Can you work these out from the model? Positions are in its coordinate system, mm. A direction names the side the tool comes from. Give positions to 0.01 mm unless a question says otherwise; leave off trailing zeros. Loops run counter-clockwise (first coordinate to the right, second up) from the corner with the lowest first, then second, coordinate; pieces in that order, holes last. Notation, with made-up numbers: M 56.25,-37 L 80.25,-37 A22 ccw 80.25,2 Z; hole C -0.5,-1 d5. An arc over 180 degrees is marked long. Answer as a JSON object with one key per item and string values.
```python
from build123d import *

# Parameters (mm, degrees)
F1_DEPTH = 120
F3_DEPTH = 1.001


# Not quite as in the source:
# - a feature names something its author has since deleted; it is built from what else it names


with BuildPart() as f1:
    # F0 (on Front) → F1 (new body)
    with BuildSketch(Plane.XZ):
        Polygon((-17.5, 6), (-17.5, 5), (-13.5, 5), (-13.5, -1), (13.5, -1), (13.5, 5), (17.5, 5), (17.5, 6), (12.5, 6), (12.5, 0), (-12.5, 0), (-12.5, 6), align=None)
    extrude(amount=F1_DEPTH)

    # F2 (on face) → F3 (cut, through all)
    with BuildSketch(Plane.XY):
        with BuildLine():
            ThreePointArc((-2.25, -28.25), (0, -30.5), (2.25, -28.25))
            Line((2.25, -28.25), (2.25, -7.75))
            ThreePointArc((2.25, -7.75), (0, -5.5), (-2.25, -7.75))
            Line((-2.25, -7.75), (-2.25, -28.25))
        make_face()
        with BuildLine():
            Line((-2.25, -43.75), (-2.25, -64.25))
            ThreePointArc((-2.25, -64.25), (0, -66.5), (2.25, -64.25))
            Line((2.25, -64.25), (2.25, -43.75))
            ThreePointArc((2.25, -43.75), (0, -41.5), (-2.25, -43.75))
        make_face()
        with BuildLine():
            Line((-2.25, -79.75), (-2.25, -100.25))
            ThreePointArc((-2.25, -100.25), (0, -102.5), (2.25, -100.25))
            Line((2.25, -100.25), (2.25, -79.75))
            ThreePointArc((2.25, -79.75), (0, -77.5), (-2.25, -79.75))
        make_face()
        with BuildLine():
            Line((-2.25, -120), (-2.25, -136.25))
            ThreePointArc((-2.25, -136.25), (0, -138.5), (2.25, -136.25))
            Line((2.25, -136.25), (2.25, -120))
            Line((2.25, -120), (-2.25, -120))
        make_face()
        with BuildLine():
            Line((-2.25, -115.75), (-2.25, -120))
            Line((-2.25, -120), (2.25, -120))
            Line((2.25, -120), (2.25, -115.75))
            ThreePointArc((2.25, -115.75), (0, -113.5), (-2.25, -115.75))
        make_face()
    extrude(amount=-F3_DEPTH, mode=Mode.SUBTRACT)


solid = f1.part
```
1) Suppose I cut it at A-A, the plane y = -26. Write out the boundary of the cut face in (x, z), and give its area (3 significant figures).
Answer list:
{"outline": "M -17.5,5 L -13.5,5 L -13.5,-1 L -2.25,-1 L -2.25,0 L -12.5,0 L -12.5,6 L -17.5,6 Z; M 2.25,-1 L 13.5,-1 L 13.5,5 L 17.5,5 L 17.5,6 L 12.5,6 L 12.5,0 L 2.25,0 Z", "area": "42.5 mm^2"}
2) Will these pins go through, and if not, where does the flat tip stop? pin 1 Ø1.2 at (x, y) = (14.5, -30.5) entering from -Z; pin 2 Ø0.5 at (y, z) = (-118.5, -0.5) entering from +X; pin 3 Ø1.8 at (y, z) = (-33.5, 3.5) entering from -X.
Answer list:
{"pin 1": "z = 5", "pin 2": "x = 13.5", "pin 3": "x = -13.5"}
3) If we mould it in two halves opening along X, with no side actions, what happens to faces 1 (the cylindrical face through (0, -113.5, -0.5)), 2 (the flat face through (15, -59, 6))? For each: +X half, -X half, draft (parallel to the pull), parting line (faces both ways), or undercut.
Answer list:
{"face 1": "undercut", "face 2": "draft"}
4) Please list where these lines run through material, in increasing order: line 1 along X through (y, z) = (-91, 4.75); line 2 along X through (y, z) = (-18.5, 5.25); line 3 along Z through (x, y) = (-8, -18.5). Write a range as from..to.
Answer list:
{"line 1": "-13.5..-12.5, 12.5..13.5", "line 2": "-17.5..-12.5, 12.5..17.5", "line 3": "-1..0"}
5) Suppose I cut it at B-B, the plane y = -110. Write out the boundary of the cut face in (x, z).
Answer list:
{"outline": "M -17.5,5 L -13.5,5 L -13.5,-1 L 13.5,-1 L 13.5,5 L 17.5,5 L 17.5,6 L 12.5,6 L 12.5,0 L -12.5,0 L -12.5,6 L -17.5,6 Z"}
6) For faces 3 (the flat face through (15, -59, 5)), 4 (the flat face through (-16, -59, 5)), 5 (the cylindrical face through (0, -66.5, -0.5)), 6 (the flat face through (-3, -59, -1)), 7 (the flat face through (-12.5, -59, 3)), which set-ups out of +Z, -Z, +X, -X, +Y, -Y let a thin tool reach every point of the face, with its end or its side?
Answer list:
{"face 3": "-Z, +X, +Y, -Y", "face 4": "-Z, -X, +Y, -Y", "face 5": "+Z, -Z", "face 6": "-Z, +X, -X, +Y, -Y", "face 7": "+Z, +Y, -Y"}
